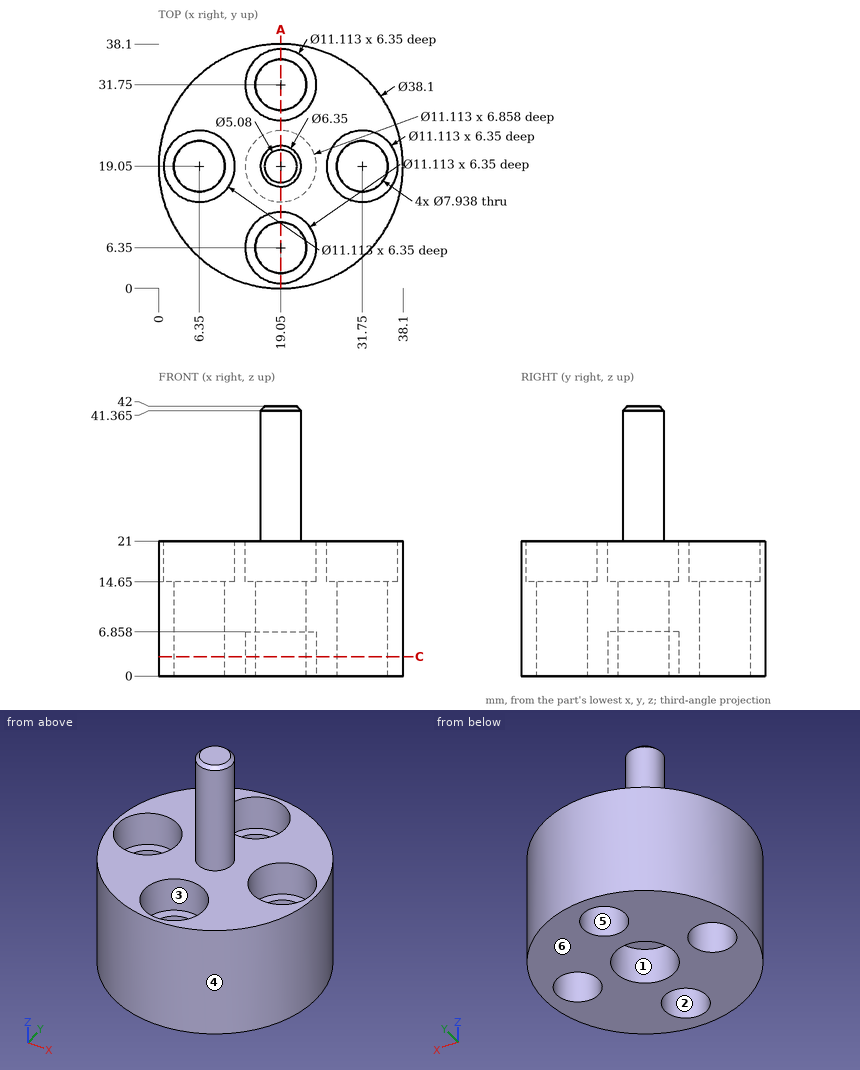
Answer from the drawing. Dimensions are ordinates in mm from the lowest x, y and z of the part. A direction names the side the tool comes from. Round coordinates to 2 decimals unless told otherwise and drop trailing zeros. Order: outer loops, then holes, each group sorted by start corner. A loop starts at its lowest first (then second) coordinate and runs counter-clockwise, first axis right, second up.
1) The part is cut by section C-C on z = 3. Write down the section's boundary in (x, y), plus the area to 3 significant figures.
2) The mould has two halves that part along X. Classify the marked faces 4, 5 and 6: released by +X, released by -X, zero draft, split by the parting line, or undercut.
3) Flat-ended cylindrical pins translate along their axes: pin 1 (7 mm diameter, centred on x = 6.35, y = 19.05, fed in from +Z); pin 2 (11.5 mm diameter, centred on x = 10.5, y = 19.5, fed in from +Z); pin 3 (5.5 mm diameter, centred on x = 6, y = 20.5, fed in from +Z); pin 4 (10 mm diameter, centred on x = 14, z = 30, fed in from -Y) (1 decimal). Find the tip coordinate at first contact, or state that the pin passes through.
4) For the marked faces 1, 2 and 3, determine the directions among +Z, -Z, +X, -X, +Y, -Y from which every point of the face is accessible in a straight line to the end or side of a thin tool.
5) Straight lines are drawn through the part: L1, parallel to X at y = 19, z = 4 (1 decimal); L2, parallel to Y at x = 19.05, z = 16.5; L3, parallel to Y at x = 19.05, z = 6. For each, find the intervals that lie inside material, in ascending order.
6) The part is cut by section A-A on x = 19.05. Give the number of separate pieces and of enclosed holes in the cut face, plus the area to 3 significant figures.
Resolved:
1. outline: circle Ø38.1 at (19.05, 19.05); hole circle Ø7.94 at (6.35, 19.05); hole circle Ø11.11 at (19.05, 19.05); hole circle Ø7.94 at (19.05, 6.35); hole circle Ø7.94 at (19.05, 31.75); hole circle Ø7.94 at (31.75, 19.05)
1. area: 845 mm2
2. face 4: split by the parting line
2. face 5: undercut
2. face 6: zero draft
3. pin 1: passes through
3. pin 2: stops at z = 41.73
3. pin 3: stops at z = 14.65
3. pin 4: stops at y = 15.9
4. face 1: -Z
4. face 2: +Z, -Z
4. face 3: +Z
5. L1: x = 0 to 2.4, 10.3 to 13.5, 24.6 to 27.8, 35.7 to 38.1
5. L2: y = 0 to 0.79, 11.91 to 26.19, 37.31 to 38.1
5. L3: y = 0 to 2.38, 10.32 to 13.49, 24.61 to 27.78, 35.72 to 38.1
6. separate pieces: 3
6. enclosed holes: 0
6. area: 483 mm2
